For this review, use the dimensioned drawing (mm, ordinates from the lowest corner) and the shaded views. A direction names the side the tool comes from. Round coordinates to 2 decimals unless told otherwise and drop trailing zeros. Write each loop counter-clockwise with the first axis right and the second up, starting at its lowest first coordinate (ties: lowest second). Pieces come first, ordered by that corner, then holes. Notation, with made-up numbers: (68, -30.5) -> (116, -30.5) arc R31 ccw to (116, 7.5) -> close; hole circle Ø8 at (26, -2.5). An arc over 180 degrees is marked (long way). Write each question's results on one line, items separated by ' | '. Start each with the question number.
Item 1: Add section B-B (x = 57.5). State the section outline as (y, z) points.
Item 2: Tool access review of the marked faces 1, 2 and 3: name each direction out of +Z, -Z, +X, -X, +Y, -Y from which nothing blocks a thin tool from reaching the whole face with its end or side.
Item 3: To check wall thickness, follow line 1 along Z through (x, y) = (32.5, 15); line 2 along Y through (x, z) = (25, 14) (1 decimal); line 3 along X through (y, z) = (76, 47). State the ranges of each line that lie inside material, in increasing order.
Item 4: Add section D-D (x = 91). State the section outline as (y, z) points.
Item 5: Clearance check with flat-ended pins moving along their axes: pin 1 (1.5 mm diameter, centred on x = 12.5, y = 82.5, fed in from +Z); pin 2 (12 mm diameter, centred on y = 15.5, z = 26.5, fed in from -X); pin 3 (12.5 mm diameter, centred on x = 96.5, z = 60, fed in from +Y). State where each tip first meets the part, or that it passes through.
Item 6: Add section C-C (z = 22). State the section outline as (x, y) points (1 decimal).
Item 7: Add section A-A (y = 60.5). State the section outline as (x, z) points (1 decimal).
Item 8: The part is to be moulded in two halves that separate along X. For the marked faces 4, 5 and 6, say which applies: +X half, -X half, draft (parallel to the pull), parting line (faces both ways), or undercut.
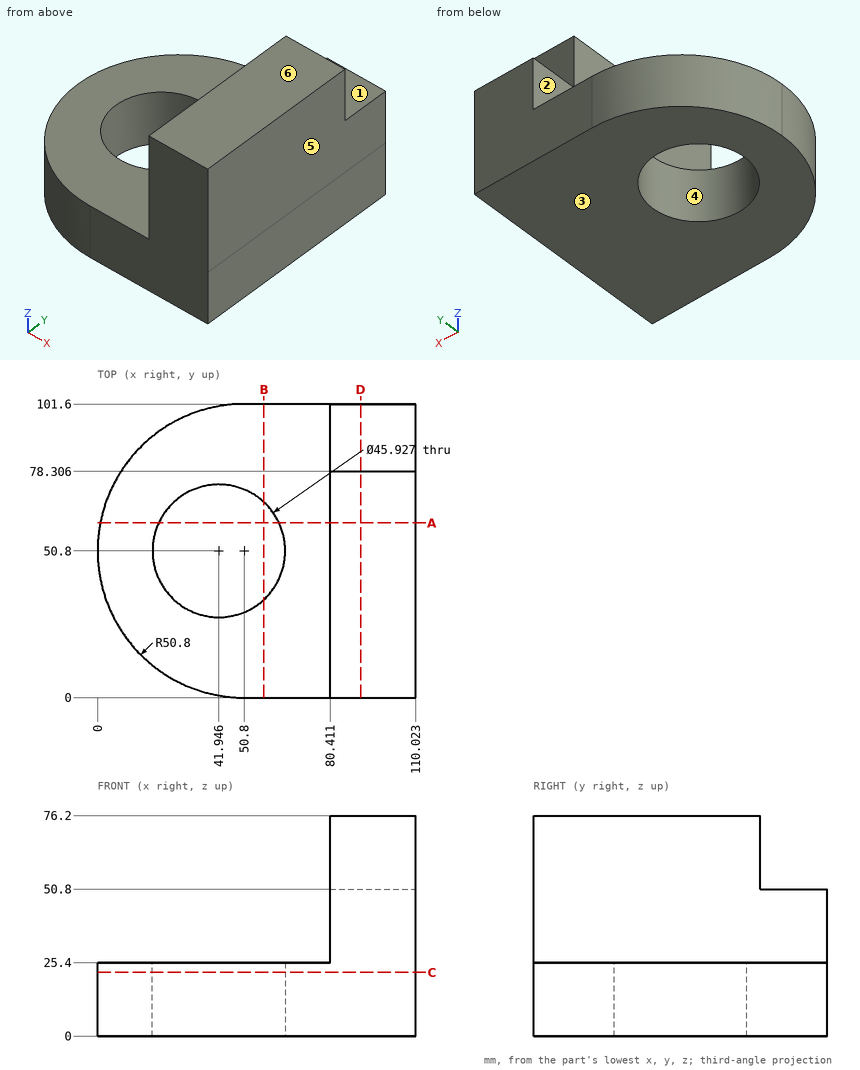
Responses:
1) outline: (0, 0) -> (33.91, 0) -> (33.91, 25.4) -> (0, 25.4) -> close; (67.69, 0) -> (101.6, 0) -> (101.6, 25.4) -> (67.69, 25.4) -> close
2) face 1: +Z, +X, -X, +Y | face 2: +Z, -X, +Y, -Y | face 3: -Z, +X, -X, +Y, -Y
3) line 1: z = 0 to 25.4 | line 2: y = 7 to 35.3, 66.3 to 94.6 | line 3: x = 80.41 to 110.02
4) outline: (0, 0) -> (101.6, 0) -> (101.6, 50.8) -> (78.31, 50.8) -> (78.31, 76.2) -> (0, 76.2) -> close
5) pin 1: stops at z = 25.4 | pin 2: stops at x = 9.37 | pin 3: stops at y = 78.31
6) outline: (50.8, 0) -> (110, 0) -> (110, 101.6) -> (50.8, 101.6) arc R50.8 ccw to start; hole circle Ø45.9 at (41.9, 50.8)
7) outline: (0.9, 0) -> (21.1, 0) -> (21.1, 25.4) -> (0.9, 25.4) -> close; (62.8, 0) -> (110, 0) -> (110, 76.2) -> (80.4, 76.2) -> (80.4, 25.4) -> (62.8, 25.4) -> close
8) face 4: undercut | face 5: +X half | face 6: draft
